The listing builds one solid part. Answer for the finished solid, in the listing's coordinates (mm). Give positions to 0.01 mm unless a question says otherwise; leave off trailing zeros. Loops run counter-clockwise (first coordinate to the right, second up) from the corner with the lowest first, then second, coordinate; pieces in that order, holes last. Notation, with made-up numbers: M 30,55.25 L 52,55.25 A29 cw 52,84.25 Z; hole C 37,85 d10. An arc over 180 degrees is marked long. Use one line per item in the form item = value. Start each with the question number.
1. The part is cut by section C-C (z = -0.5). Write down the section's boundary in (x, y).
2. The part is cut by section A-A (y = -80.5). Write down the section's boundary in (x, z), and give its area (3 significant figures).
3. The part is cut by section B-B (x = 0.9). Write down the section's boundary in (y, z) (3 decimals), and give its area (3 significant figures).
4. Straight lines are drawn through the part: line 1 (Z direction, x = 1.2, y = -33); line 2 (Z direction, x = 0.45, y = -105); line 3 (Y direction, x = 0.3, z = 68.5). For each, find the intervals that lie inside material, in ascending order. Write a range as from..to.
5. Each of these flat-tipped pins is pushed along its axis until it touches: pin 1 Ø0.6 at (x, z) = (0.5, 69) entering from +Y; pin 2 Ø0.6 at (x, z) = (0.5, 50.5) entering from -Y. Where does it stop, or does it pass through?
from build123d import *

# Parameters (mm, degrees)
BOSS_EXTRUDE1_DEPTH                          = 1.27
CUT_EXTRUDE2_REACH                           = 146.798
SKETCH7_W                                    = 9.906
SKETCH7_H                                    = 6.858
CUT_EXTRUDE3_REACH                           = 146.798
SKETCH18_R                                   = 1.143
CUT_EXTRUDE4_DEPTH                           = 2.54
CSK_FOR_M2_5_COUNTERSUNK_FLAT_HEAD_S_2_COUNT = 2
CSK_FOR_M2_5_COUNTERSUNK_FLAT_HEAD_S_2_PITCH = 31.442301831
CSK_FOR_M2_5_COUNTERSUNK_FLAT_HEAD_S_3_COUNT = 2
CSK_FOR_M2_5_COUNTERSUNK_FLAT_HEAD_S_3_PITCH = 101.252
CSK_FOR_M2_5_COUNTERSUNK_FLAT_HEAD_S_4_COUNT = 2
CSK_FOR_M2_5_COUNTERSUNK_FLAT_HEAD_S_4_PITCH = 106.021629154


with BuildPart() as part:
    # Sketch2 → Boss-Extrude1 (new body)
    with BuildSketch(Plane(origin=(0, 0, 0), x_dir=(0, 0, -1), z_dir=(1, 0, 0))):
        Polygon((36.346050031, -8.290645537), (-6.833949969, -8.290645537), (-6.833949969, 1.709354463), (-31.725949969, 1.709354463), (-31.725949969, -8.290645537), (-74.905949969, -8.290645537), (-74.905949969, -64.932645537), (-31.725949969, -64.932645537), (-31.725949969, -123.911447323), (-6.833949969, -123.911447323), (-6.833949969, -64.932645537), (36.346050031, -64.932645537), align=None)
    extrude(amount=BOSS_EXTRUDE1_DEPTH)

    # Sketch7 → Cut-Extrude2 (cut, up to next)
    with BuildSketch(Plane.ZY, mode=Mode.PRIVATE) as cut_extrude2_sk1:
        with Locations((-31.393050031, -11.719645537)):
            Rectangle(SKETCH7_W, SKETCH7_H)
    cut_extrude2_tool1 = extrude(cut_extrude2_sk1.sketch, amount=-CUT_EXTRUDE2_REACH, mode=Mode.PRIVATE) & part.part
    # Sketch7 → Cut-Extrude2 (cut, up to next)
    with BuildSketch(Plane.ZY, mode=Mode.PRIVATE) as cut_extrude2_sk2:
        with Locations((69.952949969, -11.719645537)):
            Rectangle(SKETCH7_W, SKETCH7_H)
    cut_extrude2_tool2 = extrude(cut_extrude2_sk2.sketch, amount=-CUT_EXTRUDE2_REACH, mode=Mode.PRIVATE) & part.part
    add(cut_extrude2_tool1.solids().sort_by_distance((0, -11.719646, -31.39305))[0], mode=Mode.SUBTRACT)
    add(cut_extrude2_tool2.solids().sort_by_distance((0, -11.719646, 69.95295))[0], mode=Mode.SUBTRACT)

    # Sketch10 → Cut-Extrude3 (cut, up to next)
    with BuildSketch(Plane.ZY, mode=Mode.PRIVATE) as cut_extrude3_sk1:
        with BuildLine():
            Line((21.184949969, -13.370645537), (21.184949969, -114.970645537))
            ThreePointArc((21.184949969, -114.970645537), (19.279949969, -116.875645537), (17.374949969, -114.970645537))
            Line((17.374949969, -114.970645537), (17.374949969, -13.370645537))
            ThreePointArc((17.374949969, -13.370645537), (19.279949969, -11.465645537), (21.184949969, -13.370645537))
        make_face()
    cut_extrude3_tool1 = extrude(cut_extrude3_sk1.sketch, amount=-CUT_EXTRUDE3_REACH, mode=Mode.PRIVATE) & part.part
    add(cut_extrude3_tool1.solids().sort_by_distance((0, -64.170646, 19.27995))[0], mode=Mode.SUBTRACT)

    # Sketch18 → Cut-Extrude4 (cut)
    with BuildSketch(Plane.ZY):
        with Locations((19.279949969, -5.591895537)):
            Circle(SKETCH18_R)
    extrude(amount=-CUT_EXTRUDE4_DEPTH, mode=Mode.SUBTRACT)

    # Sketch21 → CSK for M2.5 Countersunk Flat Head Screw1 (revolve, cut)
    with BuildSketch(Plane(origin=(0, -21.148645537, -31.346050031), x_dir=(0, 0, 1), z_dir=(0, 1, 0))):
        Polygon((0, 0), (0, 1.27), (1.45, 1.27), (1.45, 1.3), (2.75, 0), align=None)
    csk_for_m2_5_countersunk_flat_head_screw = revolve(axis=Axis((-6.35, -21.148645537, -31.346050031), (1, 0, 0)), mode=Mode.SUBTRACT)

    # CSK for M2.5 Countersunk Flat Head S 2: CSK for M2.5 Countersunk Flat Head Screw1 ×2
    with Locations(*[(0, -i * CSK_FOR_M2_5_COUNTERSUNK_FLAT_HEAD_S_2_PITCH, 0) for i in range(1, CSK_FOR_M2_5_COUNTERSUNK_FLAT_HEAD_S_2_COUNT)]):
        add(csk_for_m2_5_countersunk_flat_head_screw, mode=Mode.SUBTRACT)

    # CSK for M2.5 Countersunk Flat Head S 3: CSK for M2.5 Countersunk Flat Head Screw1 ×2
    with Locations(*[(0, 0, i * CSK_FOR_M2_5_COUNTERSUNK_FLAT_HEAD_S_3_PITCH) for i in range(1, CSK_FOR_M2_5_COUNTERSUNK_FLAT_HEAD_S_3_COUNT)]):
        add(csk_for_m2_5_countersunk_flat_head_screw, mode=Mode.SUBTRACT)

    # CSK for M2.5 Countersunk Flat Head S 4: CSK for M2.5 Countersunk Flat Head Screw1 ×2
    with Locations(*[Vector(0, -0.29656497529839515, 0.9550126781494905) * (i * CSK_FOR_M2_5_COUNTERSUNK_FLAT_HEAD_S_4_PITCH) for i in range(1, CSK_FOR_M2_5_COUNTERSUNK_FLAT_HEAD_S_4_COUNT)]):
        add(csk_for_m2_5_countersunk_flat_head_screw, mode=Mode.SUBTRACT)


solid = part.part
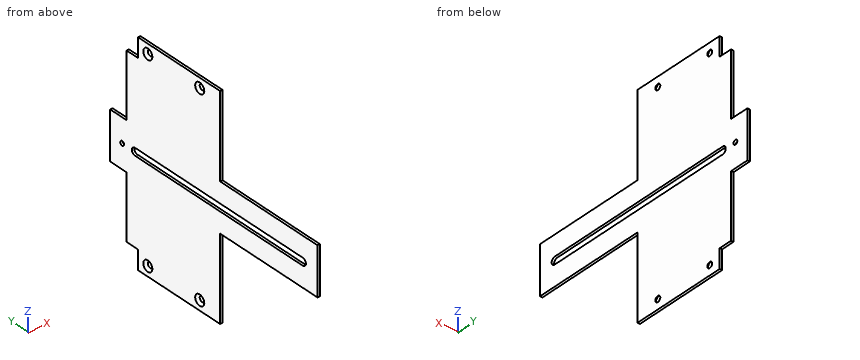
Derived:
q1.outline = M 0,-64.93 L 1.27,-64.93 L 1.27,-8.29 L 0,-8.29 Z
q2.outline = M 0,6.83 L 1.27,6.83 L 1.27,17.37 L 0,17.37 Z; M 0,21.18 L 1.27,21.18 L 1.27,31.73 L 0,31.73 Z
q2.area = 26.8 mm2
q3.outline = M -123.911,6.834 L -64.933,6.834 L -64.933,-36.346 L -15.149,-36.346 L -15.149,-26.44 L -8.291,-26.44 L -8.291,6.834 L 1.709,6.834 L 1.709,31.726 L -8.291,31.726 L -8.291,65 L -15.149,65 L -15.149,74.906 L -64.933,74.906 L -64.933,31.726 L -123.911,31.726 Z; hole M -114.971,17.375 L -13.371,17.375 A1.905 ccw -13.371,21.185 L -114.971,21.185 A1.905 ccw Z; hole C -52.591,-31.346 d3.7; hole C -52.591,69.906 d3.7; hole C -21.149,-31.346 d3.7; hole C -21.149,69.906 d3.7; hole C -5.592,19.28 d2.286
q3.area = 7,440 mm2
q4.line_1 = -36.35..17.37, 21.18..74.91
q4.line_2 = 6.83..17.37, 21.18..31.73
q4.line_3 = -64.93..-54.6, -50.58..-23.16, -19.14..-15.15
q5.pin_1 = -15.15
q5.pin_2 = -64.93
